Check sheet for the modelled part. Datum: model origin and axes. Units: mm. Face numbers are marked on the shaded views. A direction names the side the tool comes from. Coordinates: 2 decimals unless noted, no trailing zeros. Loops run counter-clockwise (first coordinate to the right, second up) from the corner with the lowest first, then second, coordinate; pieces in that order, holes last. Notation, with made-up numbers: (26, 10.25) - (43, 10.25) arc R27 cw to (43, 30.25) - close; hole circle Ø10 at (51, 54). An arc over 180 degrees is marked (long way). Use a Markdown table: item, result. Add a question column.
1) Thickness scan on line 1 (Y direction, x = -40, z = -18.5); line 2 (Z direction, x = 48.5, y = 7); line 3 (Z direction, x = 61.5, y = -67). Record the ranges inside material, lowest first.
2) Sectioned sample at C-C, the plane y = -45.5. Enter the section's corners in (x, z).
3) Go/stop test with flat-tipped pins: P1, Ø9, axis at y = 31.5, z = -17, coming from the -X side; P2, Ø9, axis at y = -67, z = -18, coming from the +X side; P3, Ø12, axis at y = 75.5, z = -13.5, coming from the -X side. Record where each tip stops, or that it passes through.
4) Sectioned sample at A-A, the plane y = 56. Enter the section's corners in (x, z).
5) Tool access check on the marked faces 4, 5, 6 and 7. Record the directions out of +Z, -Z, +X, -X, +Y, -Y that give a thin tool (end or side, any length) a straight path to the whole face; none if there is none.
6) Sectioned sample at D-D, the plane x = 8. Enter the section's corners in (y, z), then the cut area to 3 significant figures.
7) Draft check along X on the marked faces 1, 2 and 3. Enter one of: pulls with the +X half, pulls with the -X half, needs draft (parallel to the pull), parting line crosses it, or undercut.
from build123d import *

# Parameters (mm, degrees)
SALIENTE_EXTRUIR1_DEPTH = 9
CROQUIS4_W              = 92.524179437
CROQUIS4_H              = 23.337512491
CROQUIS4_R              = 1.4
CORTAR_EXTRUIR1_DEPTH   = 130.69901246
SALIENTE_EXTRUIR2_DEPTH = 18
SALIENTE_EXTRUIR3_DEPTH = 8
SALIENTE_EXTRUIR4_DEPTH = 4
CROQUIS9_W              = 22
CROQUIS9_H              = 22
SALIENTE_EXTRUIR5_DEPTH = 3


with BuildPart() as part:
    # Croquis3 → Saliente-Extruir1 (new body)
    with BuildSketch(Plane.XY):
        Polygon((-78.930426729, 27.657765941), (-78.930426729, -74.542234059), (-67.930426729, -74.542234059), (-67.930426729, -85.542234059), (-31.316827161, -85.542234059), (-31.316827161, -74.542234059), (-12.930426729, -74.542234059), (-12.930426729, -85.542234059), (23.269573271, -85.542234059), (23.269573271, -74.542234059), (41.655973703, -74.542234059), (41.655973703, -85.542234059), (78.269573271, -85.542234059), (78.269573271, -74.542234059), (89.269573271, -74.542234059), (89.269573271, 27.657765941), (78.269573271, 27.657765941), (78.269573271, 60.657765941), (67.269573271, 60.657765941), (67.269573271, 71.657765942), (56.269573271, 71.657765942), (56.269573271, 82.657765942), (34.269573271, 82.657765942), (34.269573271, 93.657765942), (-23.930426729, 93.657765942), (-23.930426729, 82.657765942), (-45.930426729, 82.657765942), (-45.930426729, 71.657765942), (-56.930426729, 71.657765942), (-56.930426729, 60.657765941), (-67.930426729, 60.657765941), (-67.930426729, 27.657765941), align=None)
    extrude(amount=-SALIENTE_EXTRUIR1_DEPTH)

    # Croquis4 → Cortar-Extruir1 (cut, through all)
    with BuildSketch(Plane(origin=(0, 0, -9), x_dir=(-1, 0, 0), z_dir=(0, 0, -1))):
        with Locations((-5.16957327, -46.12250801)):
            Rectangle(CROQUIS4_W, CROQUIS4_H)
        with Locations((-74.719573271, 24.107765941)):
            Circle(CROQUIS4_R)
        with Locations((-30.719573271, 79.107765942)):
            Circle(CROQUIS4_R)
        with Locations(Location((20.380426729, 79.107765942, 0), (0, 0, 180))):
            Circle(CROQUIS4_R)
        with Locations(Location((34.866827161, -70.992234059, 0), (0, 0, 180))):
            Circle(CROQUIS4_R)
        with Locations(Location((64.380426729, 24.107765941, 0), (0, 0, 180))):
            Circle(CROQUIS4_R)
        with Locations((-45.205973703, -70.992234059)):
            Circle(CROQUIS4_R)
    extrude(amount=-CORTAR_EXTRUIR1_DEPTH, mode=Mode.SUBTRACT)

    # Croquis5 → Saliente-Extruir2 (add)
    with BuildSketch(Plane(origin=(0, 0, -9), x_dir=(-1, 0, 0), z_dir=(0, 0, -1))):
        Polygon((71.830426729, 20.557765941), (60.830426729, 20.557765941), (60.830426729, 53.557765941), (49.830426729, 53.557765941), (49.830426729, 64.557765942), (38.830426729, 64.557765942), (38.830426729, 75.557765942), (16.830426729, 75.557765942), (16.830426729, 86.557765942), (-27.169573271, 86.557765942), (-27.169573271, 75.557765942), (-49.169573271, 75.557765942), (-49.169573271, 64.557765942), (-60.169573271, 64.557765942), (-60.169573271, 53.557765941), (-71.169573271, 53.557765941), (-71.169573271, 20.557765941), (-82.169573271, 20.557765941), (-82.169573271, -67.442234059), (-71.169573271, -67.442234059), (-71.169573271, -78.442234059), (-48.755973703, -78.442234059), (-48.755973703, -67.442234059), (-16.169573271, -67.442234059), (-16.169573271, -78.442234059), (5.830426729, -78.442234059), (5.830426729, -67.442234059), (38.416827161, -67.442234059), (38.416827161, -78.442234059), (60.830426729, -78.442234059), (60.830426729, -67.442234059), (71.830426729, -67.442234059), align=None)
        Polygon((-66.169573271, 48.557765941), (-66.169573271, 15.557765941), (-77.169573271, 15.557765941), (-77.169573271, -62.442234059), (-66.169573271, -62.442234059), (-66.169573271, -73.442234059), (-53.755973703, -73.442234059), (-53.755973703, -62.442234059), (-11.169573271, -62.442234059), (-11.169573271, -73.442234059), (0.830426729, -73.442234059), (0.830426729, -62.442234059), (43.416827161, -62.442234059), (43.416827161, -73.442234059), (55.830426729, -73.442234059), (55.830426729, -62.442234059), (66.830426729, -62.442234059), (66.830426729, 15.557765941), (55.830426729, 15.557765941), (55.830426729, 48.557765941), (44.830426729, 48.557765941), (44.830426729, 59.557765942), (33.830426729, 59.557765942), (33.830426729, 70.557765942), (11.830426729, 70.557765942), (11.830426729, 81.557765942), (-22.169573271, 81.557765942), (-22.169573271, 70.557765942), (-44.169573271, 70.557765942), (-44.169573271, 59.557765942), (-55.169573271, 59.557765942), (-55.169573271, 48.557765941), align=None, mode=Mode.SUBTRACT)
    extrude(amount=SALIENTE_EXTRUIR2_DEPTH)

    # Croquis7 → Saliente-Extruir3 (add)
    with BuildSketch(Plane(origin=(0, 0, -27), x_dir=(-1, 0, 0), z_dir=(0, 0, -1))):
        Polygon((71.830426729, -67.442234059), (71.830426729, 20.557765941), (60.830426729, 20.557765941), (60.830426729, 53.557765941), (49.830426729, 53.557765941), (49.830426729, 64.557765942), (38.830426729, 64.557765942), (38.830426729, 75.557765942), (16.830426729, 75.557765942), (16.830426729, 86.557765942), (-27.169573271, 86.557765942), (-27.169573271, 75.557765942), (-49.169573271, 75.557765942), (-49.169573271, 64.557765942), (-60.169573271, 64.557765942), (-60.169573271, 53.557765941), (-71.169573271, 53.557765941), (-71.169573271, 20.557765941), (-82.169573271, 20.557765941), (-82.169573271, -67.442234059), (-71.169573271, -67.442234059), (-71.169573271, -78.442234059), (-48.755973703, -78.442234059), (-48.755973703, -67.442234059), (-16.169573271, -67.442234059), (-16.169573271, -78.442234059), (5.830426729, -78.442234059), (5.830426729, -67.442234059), (38.416827161, -67.442234059), (38.416827161, -78.442234059), (60.830426729, -78.442234059), (60.830426729, -67.442234059), align=None)
    extrude(amount=SALIENTE_EXTRUIR3_DEPTH)

    # Croquis8 → Saliente-Extruir4 (add)
    with BuildSketch(Plane(origin=(0, 0, -35), x_dir=(-1, 0, 0), z_dir=(0, 0, -1))):
        Polygon((-71.169573271, 20.557765941), (-71.169573271, 9.557765941), (-60.169573271, 9.557765941), (-60.169573271, -1.442234059), (-38.169573271, -1.442234059), (-38.169573271, 9.557765941), (-27.169573271, 9.557765941), (-27.169573271, 20.557765941), (-27.169573271, 42.557765941), (-38.169573271, 42.557765941), (-38.169573271, 53.557765941), (-60.169573271, 53.557765941), (-60.169573271, 42.557765941), (-71.169573271, 42.557765941), align=None)
        Polygon((38.830426729, 20.557765941), (38.830426729, 9.557765941), (27.830426729, 9.557765941), (27.830426729, -1.442234059), (5.830426729, -1.442234059), (5.830426729, 9.557765941), (-5.169573271, 9.557765941), (-5.169573271, 20.557765941), (-5.169573271, 42.557765941), (5.830426729, 42.557765941), (5.830426729, 53.557765941), (27.830426729, 53.557765941), (27.830426729, 42.557765941), (38.830426729, 42.557765941), align=None)
    extrude(amount=SALIENTE_EXTRUIR4_DEPTH)

    # Croquis9 → Saliente-Extruir5 (add)
    with BuildSketch(Plane(origin=(0, 0, -39), x_dir=(-1, 0, 0), z_dir=(0, 0, -1))):
        with Locations((-60.169573271, 20.557765941)):
            Rectangle(CROQUIS9_W, CROQUIS9_H)
        with Locations((5.830426729, 20.557765941)):
            Rectangle(CROQUIS9_W, CROQUIS9_H)
    extrude(amount=SALIENTE_EXTRUIR5_DEPTH)


solid = part.part
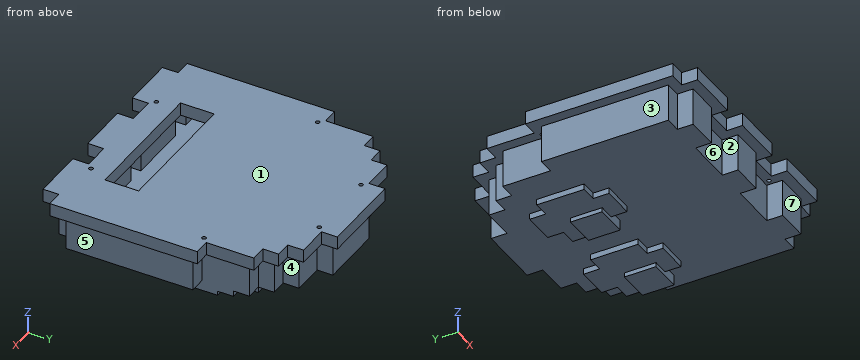
Solved:
| question | item | result |
|---|---|---|
| 1 | line 1 | y = -78.44 to -62.44, 59.56 to 64.56 |
| 1 | line 2 | z = -39 to -27, -9 to 0 |
| 1 | line 3 | z = -35 to -27, -9 to 0 |
| 2 | outline | (-78.93, -9) - (-71.83, -9) - (-71.83, -35) - (82.17, -35) - (82.17, -9) - (89.27, -9) - (89.27, 0) - (51.43, 0) - (51.43, -9) - (77.17, -9) - (77.17, -27) - (-66.83, -27) - (-66.83, -9) - (-41.09, -9) - (-41.09, 0) - (-78.93, 0) - close |
| 3 | P1 | stops at x = -60.83 |
| 3 | P2 | stops at x = 82.17 |
| 3 | P3 | stops at x = -56.93 |
| 4 | outline | (-67.93, -9) - (-49.83, -9) - (-49.83, -35) - (60.17, -35) - (60.17, -9) - (78.27, -9) - (78.27, 0) - (-67.93, 0) - close; hole (-44.83, -27) - (55.17, -27) - (55.17, -9) - (-44.83, -9) - close |
| 5 | face 4 | -Z, +X, +Y |
| 5 | face 5 | -Z, +X, +Y, -Y |
| 5 | face 6 | -Z, -Y |
| 5 | face 7 | -Z, +X, -X, -Y |
| 6 | outline | (-85.54, -9) - (-78.44, -9) - (-78.44, -35) - (86.56, -35) - (86.56, -9) - (93.66, -9) - (93.66, 0) - (-34.45, 0) - (-34.45, -9) - (81.56, -9) - (81.56, -27) - (-73.44, -27) - (-73.44, -9) - (-57.79, -9) - (-57.79, 0) - (-85.54, 0) - close |
| 6 | area | 2,900 mm2 |
| 7 | face 1 | needs draft |
| 7 | face 2 | undercut |
| 7 | face 3 | pulls with the -X half |
